The listing builds one solid part. Answer for the finished solid, in the listing's coordinates (mm). Face numbers are marked on the shaded views. A direction names the side the tool comes from. Round coordinates to 2 decimals unless told otherwise and drop trailing zeros. Write each loop counter-clockwise with the first axis right and the second up, starting at its lowest first coordinate (ties: lowest second). Pieces come first, ordered by that corner, then holes. Notation, with made-up numbers: (43, 16.25) - (65, 16.25) arc R16 ccw to (65, 29.25) - close; hole circle Ø2 at (71.25, -9.5). An arc over 180 degrees is marked (long way). Return JSON: item names as keys, results as strings. Group by question number.
(1) Determine the mould class of the marked faces 1, 2, 3 and 4 for opening direction Y: +Y half, -Y half, draft (parallel to the pull), parting line (faces both ways), or undercut.
(2) Section A-A, the plane y = 0.5 is taken. Write down the section's boundary in (x, z), then the cut area to 3 significant figures.
(3) Find the intervals of material crossed by line 1 along X through (y, z) = (-0.5, 0); line 2 along Y through (x, z) = (-4.5, -5); line 3 along X through (y, z) = (2, -2.5), in increasing order. Write a range as [from, to].
(4) Which of the six approach directions +Z, -Z, +X, -X, +Y, -Y give full straight-line access (tool end or side, diameter ignored) to the marked faces 5, 6 and 7?
(5) Section D-D, the plane y = 8.5 is taken. Write down the section's boundary in (x, z), then the cut area to 3 significant figures.
(6) Each of these flat-tipped pins is pushed along its axis until it touches: pin 1 (4 mm diameter, centred on y = 8.5, z = -2.5, fed in from +X); pin 2 (1 mm diameter, centred on y = 1.5, z = 5, fed in from +X); pin 3 (5 mm diameter, centred on y = 6, z = -1.5, fed in from -X). Where does it stop, or does it pass through?
(7) Section B-B, the plane x = -7.25 is taken. Write down the section's boundary in (y, z).
(8) Section C-C, the plane z = 1.5 is taken. Write down the section's boundary in (x, y).
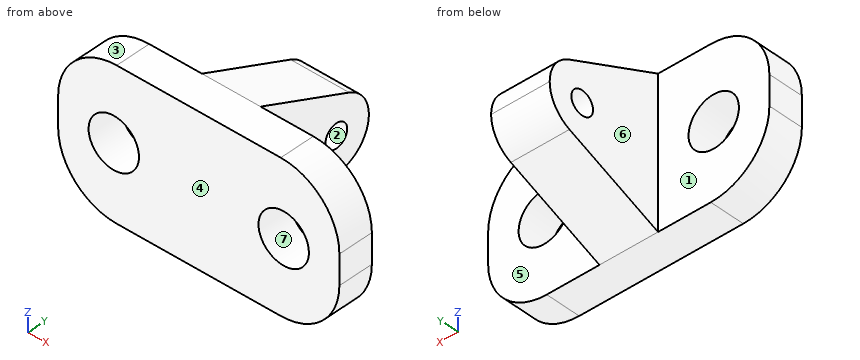
```python
from build123d import *

# Parameters (mm, degrees)
SKETCH1_R               = 2.15
BOSS_EXTRUDE1_DEPTH     = 1.5
SKETCH3_W               = 5
SKETCH3_H               = 10
BOSS_EXTRUDE3_DEPTH     = 12.5
CUT_EXTRUDE1_DEPTH      = 20.533624856
CUT_EXTRUDE1_DEPTH_BACK = 20.533624856
SKETCH4_R               = 1


with BuildPart() as part:
    # Sketch1 → Boss-Extrude1 (new, symmetric)
    with BuildSketch(Plane(origin=(0, 0, 0), x_dir=(1, 0, 0), z_dir=(0, 1, 0))):
        with BuildLine():
            Line((-7, -6.25), (7, -6.25))
            ThreePointArc((7, -6.25), (10.535533906, -4.785533906), (12, -1.25))
            Line((12, -1.25), (12, 1.25))
            ThreePointArc((12, 1.25), (10.535533906, 4.785533906), (7, 6.25))
            Line((7, 6.25), (-7, 6.25))
            ThreePointArc((-7, 6.25), (-10.535533906, 4.785533906), (-12, 1.25))
            Line((-12, 1.25), (-12, -1.25))
            ThreePointArc((-12, -1.25), (-10.535533906, -4.785533906), (-7, -6.25))
        make_face()
        with Locations(Location((-7.25, 0, 0), (0, 0, 270))):
            Circle(SKETCH1_R, mode=Mode.SUBTRACT)
        with Locations(Location((7.25, 0, 0), (0, 0, 270))):
            Circle(SKETCH1_R, mode=Mode.SUBTRACT)
    extrude(amount=BOSS_EXTRUDE1_DEPTH, both=True)

    # Sketch3 → Boss-Extrude3 (add)
    with BuildSketch(Plane.XY.offset(6.25)):
        with Locations((0, 6.5)):
            Rectangle(SKETCH3_W, SKETCH3_H)
    extrude(amount=-BOSS_EXTRUDE3_DEPTH)

    # Sketch4 → Cut-Extrude1 (cut, two sides: drawn at the far end of the back side and taken through both)
    with BuildSketch(Plane.ZY.offset(2.5).offset(-CUT_EXTRUDE1_DEPTH_BACK)):
        with BuildLine():
            Line((-6.25, 1.5), (-2.759130187, 9.677794809))
            ThreePointArc((-2.759130187, 9.677794809), (-1.653271843, 11.003336217), (0, 11.5))
            Line((0, 11.5), (-6.25, 11.5))
            Line((-6.25, 11.5), (-6.25, 1.5))
        make_face()
        with BuildLine():
            Line((6.25, 11.5), (0, 11.5))
            ThreePointArc((0, 11.5), (1.653271843, 11.003336217), (2.759130187, 9.677794809))
            Line((2.759130187, 9.677794809), (6.25, 1.5))
            Line((6.25, 1.5), (6.25, 11.5))
        make_face()
        with Locations((0, 8.5)):
            Circle(SKETCH4_R)
    extrude(amount=CUT_EXTRUDE1_DEPTH + CUT_EXTRUDE1_DEPTH_BACK, mode=Mode.SUBTRACT)


solid = part.part
```
Working result:
{
 "1": {"face 1": "+Y half", "face 2": "undercut", "face 3": "draft", "face 4": "-Y half"},
 "2": {"outline": "(-12, -1.25) arc R5 ccw to (-7, -6.25) - (7, -6.25) arc R5 ccw to (12, -1.25) - (12, 1.25) arc R5 ccw to (7, 6.25) - (-7, 6.25) arc R5 ccw to (-12, 1.25) - close; hole circle Ø4.3 at (-7.25, 0); hole circle Ø4.3 at (7.25, 0)", "area": "249 mm^2"},
 "3": {"line 1": "x = [-12, -9.4], [-5.1, 5.1], [9.4, 12]", "line 2": "y = [-1.5, 1.5]", "line 3": "x = [-2.5, 2.5]"},
 "4": {"face 5": "+Z, -Z, +X, +Y", "face 6": "+Z, -Z, -X, +Y", "face 7": "+Y, -Y"},
 "5": {"outline": "(-2.5, -3.26) - (2.5, -3.26) - (2.5, -1) - (-2.5, -1) - close; (-2.5, 1) - (2.5, 1) - (2.5, 3.26) - (-2.5, 3.26) - close", "area": "22.6 mm^2"},
 "6": {"pin 1": "stops at x = 2.5", "pin 2": "stops at x = 10.8", "pin 3": "stops at x = -2.5"},
 "7": {"outline": "(-1.5, -6.24) - (1.5, -6.24) - (1.5, -2.15) - (-1.5, -2.15) - close; (-1.5, 2.15) - (1.5, 2.15) - (1.5, 6.24) - (-1.5, 6.24) - close"},
 "8": {"outline": "(-11.99, -1.5) - (-8.79, -1.5) - (-8.79, 1.5) - (-11.99, 1.5) - close; (-5.71, -1.5) - (5.71, -1.5) - (5.71, 1.5) - (2.5, 1.5) - (2.5, 11.1) - (-2.5, 11.1) - (-2.5, 1.5) - (-5.71, 1.5) - close; (8.79, -1.5) - (11.99, -1.5) - (11.99, 1.5) - (8.79, 1.5) - close"}
}
